```python
from build123d import *

# Parameters (mm, degrees)
F2_DEPTH = 7.62
F1_R     = 8.475319
F3_DEPTH = 73.914


with BuildPart() as f2:
    # F0 (on Top) → F2 (new body)
    with BuildSketch(Plane.XY):
        Polygon((-10.998523, 6.35), (0, 0), (0, 50.8), align=None)
        Polygon((-10.998523, 6.35), (-43.994091, -25.4), (0, 0), align=None)
        Polygon((0, 0), (-43.994091, -25.4), (0, -12.7), align=None)
        Polygon((43.994091, -25.4), (0, 0), (0, -12.7), align=None)
        Polygon((0, 50.8), (0, 0), (10.998523, 6.35), align=None)
        Polygon((10.998523, 6.35), (0, 0), (43.994091, -25.4), align=None)
    extrude(amount=F2_DEPTH)

    # F1 (on Top) → F3 (cut)
    with BuildSketch(Plane.XY):
        Circle(F1_R)
    extrude(amount=F3_DEPTH, mode=Mode.SUBTRACT)


solid = f2.part
```
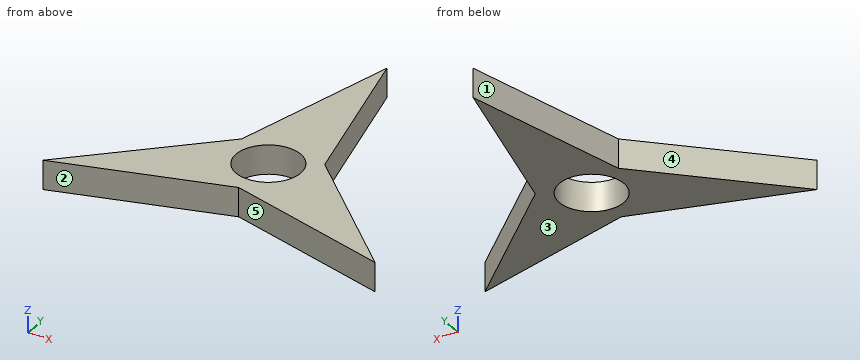
Could you check a few things on this model? Use its own coordinates, in mm. Face numbers are marked on the shaded views. A direction names the side the tool comes from. Round coordinates to 2 decimals unless told otherwise and drop trailing zeros. Loops run counter-clockwise (first coordinate to the right, second up) from the corner with the lowest first, then second, coordinate; pieces in that order, holes last. Notation, with made-up numbers: M -24.75,-26.75 L 22.25,-26.75 A10 ccw 22.25,-7.75 Z; hole C 79.25,-17 d10. An arc over 180 degrees is marked long. Put each result on its own line as item: value.
Q1. Thinking about a two-plate mould opening in X: for the marked faces 3, 4 and 5, which applies, released by +X, released by -X, zero draft, split by the parting line, or undercut?
Check result:
face 3: zero draft
face 4: released by -X
face 5: undercut
Q2. Imagine slicing it at C-C (x = -19.5). Write out the boundary of the cut face in (y, z).
Check result:
outline: M -18.33,0 L -1.83,0 L -1.83,7.62 L -18.33,7.62 Z
Q3. Imagine slicing it at A-A (z = 1.25). Write out the boundary of the cut face in (x, y).
Check result:
outline: M -43.99,-25.4 L 0,-12.7 L 43.99,-25.4 L 11,6.35 L 0,50.8 L -11,6.35 Z; hole C 0,0 d16.95
Q4. For pin 1 (2 mm diameter, centred on y = 0.5, z = 1.5, fed in from -X); pin 2 (2 mm diameter, centred on y = 6, z = 3.5, fed in from -X); pin 3 (1 mm diameter, centred on y = 36, z = 4, fed in from +X), each with a flat end and sliding along its axis, tell me the tip position at first contact or that it passes through.
Check result:
pin 1: x = -18.12
pin 2: x = -12.4
pin 3: x = 3.79
Q5. Imagine slicing it at D-D (y = 17.5). Write out the boundary of the cut face in (x, z).
Check result:
outline: M -8.24,0 L 8.24,0 L 8.24,7.62 L -8.24,7.62 Z
Q6. On a 3-axis mill with a long thin cutter (end or side, diameter ignored), from which of +Z, -Z, +X, -X, +Y, -Y can I reach the whole of each face in a straight line? I mean the marked faces 1 and 2. Say none if no direction works.
Check result:
face 1: +Z, -Z, -X, +Y
face 2: +Z, -Z, -Y
Q7. I need wall thicknesses on probe 1 along X at (y, z) = (0, 2.75); probe 2 along X at (y, z) = (2.5, 6.25); probe 3 along Y at (x, z) = (-13, 1.75). Which ranges of each line are inside material? Lowest first, please.
Check result:
probe 1: -17.6 to -8.48, 8.48 to 17.6
probe 2: -15 to -8.1, 8.1 to 15
probe 3: -16.45 to 4.42
Q8. Imagine slicing it at B-B (y = 0). Write out the boundary of the cut face in (x, z), then the cut area to 3 significant figures.
Check result:
outline: M -17.6,0 L -8.48,0 L -8.48,7.62 L -17.6,7.62 Z; M 8.48,0 L 17.6,0 L 17.6,7.62 L 8.48,7.62 Z
area: 139 mm2
